```python
from build123d import *

# Parameters (mm, degrees)
SKETCH_1_R      = 0.75
SKETCH_1_W      = 3
SKETCH_1_H      = 10
EXTRUDE_1_DEPTH = 3


with BuildPart() as part:
    # 草图1 → 凸台-拉伸1 (new body)
    with BuildSketch(Plane.XY):
        Polygon((-43.5, -20), (-4.599481492, -20), (-4.599481492, -23), (5.400518508, -23), (5.400518508, -20), (43.5, -20), (43.5, -23), (53.5, -23), (53.5, -20), (77, -20), (77, 20), (53.5, 20), (53.5, 23), (43.5, 23), (43.5, 20), (5.400518508, 20), (5.400518508, 23), (-4.599481492, 23), (-4.599481492, 20), (-43.5, 20), (-43.5, 23), (-53.5, 23), (-53.5, 20), (-77, 20), (-77, -20), (-53.5, -20), (-53.5, -23), (-43.5, -23), align=None)
        with Locations((-54.4, -14)):
            Circle(SKETCH_1_R, mode=Mode.SUBTRACT)
        with Locations(Location((-54.4, 14, 0), (0, 0, 180))):
            Circle(SKETCH_1_R, mode=Mode.SUBTRACT)
        with Locations(Location((-42, -14, 0), (0, 0, 180))):
            Circle(SKETCH_1_R, mode=Mode.SUBTRACT)
        with Locations((-42, 14)):
            Circle(SKETCH_1_R, mode=Mode.SUBTRACT)
        with Locations((42, -14)):
            Circle(SKETCH_1_R, mode=Mode.SUBTRACT)
        with Locations(Location((54.4, -14, 0), (0, 0, 180))):
            Circle(SKETCH_1_R, mode=Mode.SUBTRACT)
        with Locations((54.4, 14)):
            Circle(SKETCH_1_R, mode=Mode.SUBTRACT)
        with Locations(Location((42, 14, 0), (0, 0, 180))):
            Circle(SKETCH_1_R, mode=Mode.SUBTRACT)
        with Locations((-72.5, 0)):
            Rectangle(SKETCH_1_W, SKETCH_1_H, mode=Mode.SUBTRACT)
        with Locations((72.5, 0)):
            Rectangle(SKETCH_1_W, SKETCH_1_H, mode=Mode.SUBTRACT)
        Polygon((-60.5, 11.5), (-54.05, 11.5), (-54.05, 12.40163795), (-52.05, 12.40163795), (-52.05, 11.5), (-44.35, 11.5), (-44.35, 12.40163795), (-42.35, 12.40163795), (-42.35, 11.5), (-35.9, 11.5), (-35.9, -11.5), (-60.5, -11.5), align=None, mode=Mode.SUBTRACT)
        Polygon((52.05, 11.5), (52.05, 12.40163795), (54.05, 12.40163795), (54.05, 11.5), (60.5, 11.5), (60.5, -11.5), (35.9, -11.5), (35.9, 11.5), (42.35, 11.5), (42.35, 12.40163795), (44.35, 12.40163795), (44.35, 11.5), align=None, mode=Mode.SUBTRACT)
    extrude(amount=EXTRUDE_1_DEPTH)


solid = part.part
```
Here's how the part is built. I have some questions about the finished solid (model axes, mm). A direction names the side the tool comes from. Coordinates: 2 decimals unless noted, no trailing zeros. Order: outer loops, then holes, each group sorted by start corner. A loop starts at its lowest first (then second) coordinate and runs counter-clockwise, first axis right, second up.
1) Imagine slicing it at C-C on x = -67. List the corners of the cut face in (y, z) for me.
2) Imagine slicing it at B-B on z = 2.5. State how many separate pieces and enclosed holes the cut face has, and give its area (3 significant figures).
3) I need wall thicknesses on line 1 (Y direction, x = -42, z = 1.45); line 2 (X direction, y = -9, z = 2.7); line 3 (X direction, y = -3.5, z = 1). Which ranges of each line are inside material? Lowest first, please.
4) Will these pins go through, and if not, where does the flat tip stop? pin 1 (1.5 mm diameter, centred on y = -22, z = 1.5, fed in from -X); pin 2 (1.7 mm diameter, centred on x = -54.4, y = -14, fed in from +Z); pin 3 (1.5 mm diameter, centred on x = -59.5, z = 1, fed in from -Y).
5) We'd pull the mould along X, two halves only. Please class faces 1 (the face through (-53.5, 22, 1)), 2 (the face through (49, 23, 1)), 3 (the face through (-48, 11.5, 1)), 4 (the face through (53.5, -22, 1)): +X half, -X half, draft (parallel to the pull), parting line (faces both ways), or undercut.
6) Imagine slicing it at A-A on y = 9. List the corners of the cut face in (x, z) for me, and give its area (3 significant figures).
7) Which directions (+Z, -Z, +X, -X, +Y, -Y) give clear straight access to the entire face, cutting with the end or side of a thin tool? Please do faces 5 (the face through (65, -20, 1)), 6 (the face through (-57, 11.5, 1)), 7 (the face through (5.401, 21, 1)), 8 (the face through (-24, -20, 1)).
Response values:
1. outline: (-20, 0) - (20, 0) - (20, 3) - (-20, 3) - close
2. separate pieces: 1
2. enclosed holes: 12
2. area: 5,130 mm2
3. line 1: y = -20 to -14.75, -13.25 to -11.5, 11.5 to 13.25, 14.75 to 20
3. line 2: x = -77 to -60.5, -35.9 to 35.9, 60.5 to 77
3. line 3: x = -77 to -74, -71 to -60.5, -35.9 to 35.9, 60.5 to 71, 74 to 77
4. pin 1: stops at x = -53.5
4. pin 2: stops at z = 3
4. pin 3: stops at y = -20
5. face 1: -X half
5. face 2: draft
5. face 3: undercut
5. face 4: +X half
6. outline: (-77, 0) - (-60.5, 0) - (-60.5, 3) - (-77, 3) - close; (-35.9, 0) - (35.9, 0) - (35.9, 3) - (-35.9, 3) - close; (60.5, 0) - (77, 0) - (77, 3) - (60.5, 3) - close
6. area: 314 mm2
7. face 5: +Z, -Z, +X, -Y
7. face 6: +Z, -Z
7. face 7: +Z, -Z, +Y
7. face 8: +Z, -Z, -Y
